Work out the finished part from the listing and answer in its coordinate system (mm). A direction names the side the tool comes from. Round coordinates to 2 decimals unless told otherwise and drop trailing zeros. Order: outer loops, then holes, each group sorted by start corner. A loop starts at its lowest first (then second) coordinate and runs counter-clockwise, first axis right, second up. Notation, with made-up numbers: (-35.75, 62.25) - (-23.75, 62.25) arc R23 ccw to (-23.75, 96.25) - close; hole circle Ø5 at (7, 11.25). An arc over 180 degrees is marked (long way). Use CSV: the item, a comma, the result in double quotes.
from build123d import *

# Parameters (mm, degrees)
F0_W      = 85
F0_H      = 80
F1_DEPTH  = 1.6
F2_W      = 7.6
F2_H      = 30.6
F3_DEPTH  = 10
F5_D      = 3
F7_D      = 3
F9_D      = 3
F11_D     = 3
F14_W     = 80.6
F14_H     = 7.6
F15_DEPTH = 10


with BuildPart() as f1:
    # F0 (on Top) → F1 (new body)
    with BuildSketch(Plane.XY):
        Rectangle(F0_W, F0_H)
    extrude(amount=F1_DEPTH)

    # F2 (on face) → F3 (join)
    with BuildSketch(Plane.XY.offset(1.6)):
        with Locations((-35.95, -3.3)):
            Rectangle(F2_W, F2_H)
    extrude(amount=F3_DEPTH)

    # F5 (through all)
    with Locations(Plane.XY.offset(1.6)):
        with Locations((-38, 26)):
            Hole(F5_D / 2)

    # F7 (through all)
    with Locations(Plane(origin=(0, 0, 0), x_dir=(1, 0, 0), z_dir=(0, 0, -1))):
        with Locations((38, -26)):
            Hole(F7_D / 2)

    # F9 (through all)
    with Locations(Plane.XY.offset(1.6)):
        with Locations((38, -35.5)):
            Hole(F9_D / 2)

    # F11 (through all)
    with Locations(Plane.XY.offset(1.6)):
        with Locations((-38, -35.5)):
            Hole(F11_D / 2)


with BuildPart() as f12_1:
    # F12: copy of F1
    add(f1.part)


with BuildPart() as f1_1:
    add(f1.part)

    # F14 (on face) → F15 (join)
    with BuildSketch(Plane.XY.offset(1.6)):
        with Locations((0.8, 36.2)):
            Rectangle(F14_W, F14_H)
    extrude(amount=F15_DEPTH)


solid = f1_1.part
(1) Find section D-D (x = -38). Determine the outline of the cut face in (y, z), and give its area (3 significant figures).
Findings below:
outline,"(-40, 0) - (-37, 0) - (-37, 1.6) - (-40, 1.6) - close; (-34, 0) - (24.5, 0) - (24.5, 1.6) - (12, 1.6) - (12, 11.6) - (-18.6, 11.6) - (-18.6, 1.6) - (-34, 1.6) - close; (27.5, 0) - (40, 0) - (40, 11.6) - (32.4, 11.6) - (32.4, 1.6) - (27.5, 1.6) - close"
area,"500 mm²"
(2) Each of these flat-tipped pins is pushed along its axis until it touches: pin 1 (2.5 mm diameter, centred on y = 38, z = 7, fed in from -X); pin 2 (6 mm diameter, centred on x = 23, y = 11.5, fed in from +Z); pin 3 (2.5 mm diameter, centred on x = -34.5, z = 8.5, fed in from -Y). Where does it stop, or does it pass through?
Findings below:
pin 1,"stops at x = -39.5"
pin 2,"stops at z = 1.6"
pin 3,"stops at y = -18.6"
(3) Find section C-C (y = 26). Determine the outline of the cut face in (x, z).
Findings below:
outline,"(-42.5, 0) - (-39.5, 0) - (-39.5, 1.6) - (-42.5, 1.6) - close; (-36.5, 0) - (36.5, 0) - (36.5, 1.6) - (-36.5, 1.6) - close; (39.5, 0) - (42.5, 0) - (42.5, 1.6) - (39.5, 1.6) - close"
(4) Find section A-A (x = 38). Determine the outline of the cut face in (y, z).
Findings below:
outline,"(-40, 0) - (-37, 0) - (-37, 1.6) - (-40, 1.6) - close; (-34, 0) - (24.5, 0) - (24.5, 1.6) - (-34, 1.6) - close; (27.5, 0) - (40, 0) - (40, 11.6) - (32.4, 11.6) - (32.4, 1.6) - (27.5, 1.6) - close"
(5) For faces 1 (the flat face through (-39.75, -4, 7)), 2 (the flat face through (-36, -18.6, 7)), 3 (the flat face through (41.1, 36, 7)), 4 (the flat face through (-32.15, -4, 7)), determine the directions among +Z, -Z, +X, -X, +Y, -Y from which every point of the face is accessible in a straight line to the end or side of a thin tool.
Findings below:
face 1,"+Z, -X, +Y, -Y"
face 2,"+Z, +X, -X, -Y"
face 3,"+Z, +X, +Y, -Y"
face 4,"+Z, +X, -Y"
(6) Find the intervals of material crossed by L1, parallel to Y at x = 38, z = 0.7; L2, parallel to Y at x = -36.5, z = 3.5; L3, parallel to Y at x = 37, z = 1.75, in increasing order. Write a range as from..to.
Findings below:
L1,"y = -40..-37, -34..24.5, 27.5..40"
L2,"y = -18.6..12, 32.4..40"
L3,"y = 32.4..40"
(7) Find section B-B (z = 3.75). Determine the outline of the cut face in (x, y), and give its area (3 significant figures).
Findings below:
outline,"(-39.75, -18.6) - (-32.15, -18.6) - (-32.15, 12) - (-39.75, 12) - close; (-39.5, 32.4) - (41.1, 32.4) - (41.1, 40) - (-39.5, 40) - close"
area,"845 mm²"
(8) The mould has two halves that part along Y. Classify faces 5 (the flat face through (-39.5, 36, 7)), 6 (the flat face through (-36, 12, 7)), 7 (the flat face through (-1, 40, 6)): released by +Y, released by -Y, zero draft, split by the parting line, or undercut.
Findings below:
face 5,"zero draft"
face 6,"undercut"
face 7,"released by +Y"
